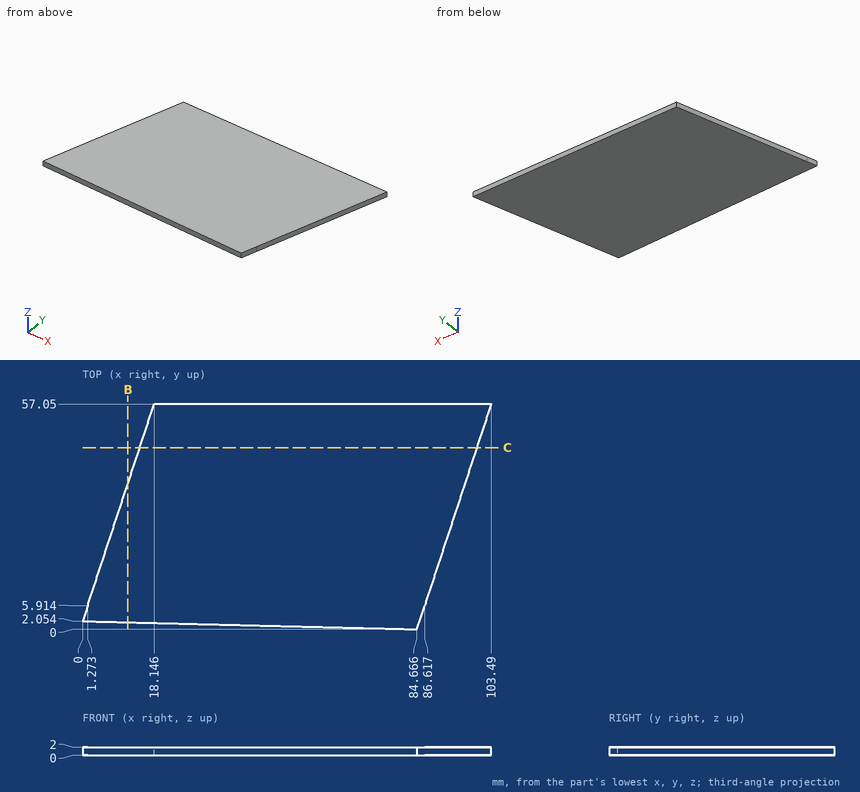
Can you work these out from the drawing? Everything is in mm from the part's minimum corner. Round coordinates to 2 decimals unless told otherwise and drop trailing zeros. Write each loop counter-clockwise with the first axis right and the second up, starting at its lowest first coordinate (ties: lowest second). Pieces come first, ordered by that corner, then holes. Notation, with made-up numbers: (-31.5, 23) - (-20.5, 23) arc R31 cw to (-20.5, 52) - close; hole circle Ø9 at (-3, -12.75). An arc over 180 degrees is marked (long way). Write each question's results on one line, items separated by ' | '. Start each with the question number.
1) Please list where these lines run through material, in increasing order: line 1 (Y direction, x = 32, z = 1); line 2 (X direction, y = 38, z = 1.35) (1 decimal); line 3 (X direction, y = 43, z = 0.6) (1 decimal).
2) Suppose I cut it at B-B (x = 11.5). List the corners of the cut face in (y, z) for me (1 decimal).
3) Suppose I cut it at C-C (y = 46). List the corners of the cut face in (x, z) for me, and give its area (3 significant figures).
4) For pin 1 Ø3 at (x, y) = (70, 12.5) entering from -Z, with a flat end and sliding along its axis, tell me the tip position at first contact or that it passes through.
Here are the results:
1) line 1: y = 1.28 to 57.05 | line 2: x = 11.9 to 97.2 | line 3: x = 13.5 to 98.9
2) outline: (1.8, 0) - (36.9, 0) - (36.9, 2) - (1.8, 2) - close
3) outline: (14.5, 0) - (99.84, 0) - (99.84, 2) - (14.5, 2) - close | area: 171 mm2
4) pin 1: stops at z = 0
